Verification items for the finished model (mm, model axes). A direction names the side the tool comes from. Round coordinates to 2 decimals unless told otherwise and drop trailing zeros. Order: outer loops, then holes, each group sorted by start corner. A loop starts at its lowest first (then second) coordinate and runs counter-clockwise, first axis right, second up. Notation, with made-up numbers: (-39.75, 18) -> (-26.75, 18) arc R21 ccw to (-26.75, 22) -> close; hole circle Ø6 at (14, 53). An arc over 180 degrees is marked (long way). Return JSON: item names as keys, results as strings. Group by question number.
1) Tool access check on faces 1 (the flat face through (7, 0, 8)), 2 (the flat face through (-12.3, -3.7, 9)), 3 (the flat face through (-6, 3, 14)). Record the directions out of +Z, -Z, +X, -X, +Y, -Y that give a thin tool (end or side, any length) a straight path to the whole face; none if there is none.
2) Draft check along Y on faces 4 (the cylindrical face through (-4.769, -21.477, 6.902)), 5 (the cylindrical face through (-1.398, -6.297, 11.042)), 6 (the flat face through (-8.3, -16.2, 14)). Enter one of: pulls with the +Y half, pulls with the -Y half, needs draft (parallel to the pull), parting line crosses it, or undercut.
3) Section check A-A on x = 0. Enter the section's corners in (y, z).
4) Scan lines: L1, parallel to Y at x = 0, z = 10.7; L2, parallel to Y at x = 0, z = 2.5; L3, parallel to X at y = -9.5, z = 9.5. Record each from-to range of solid material in increasing order.
5) Depth check by flat-ended pin: pin 1 (3 mm diameter, centred on x = 1, z = 2, fed in from -Y); pin 2 (1 mm diameter, centred on x = -5.5, y = -12, fed in from +Z); pin 3 (4 mm diameter, centred on x = -2.5, y = -6, fed in from -Z). Enter the tip coordinate at first touch or a pass-through.
6) Section check C-C on z = 11.25. Enter the section's corners in (x, y).
7) Section check D-D on y = -14.5. Enter the section's corners in (x, z).
```python
from build123d import *

# Parameters (mm, degrees)
SKETCH_R        = 22
PAD_DEPTH       = 14
SKETCH001_R     = 18
POCKET_DEPTH    = 5
SKETCH002_R     = 12.6
PAD001_DEPTH    = 5
SKETCH003_R     = 6.45
POCKET001_DEPTH = 14.001
SKETCH004_R     = 16.2
POCKET002_DEPTH = 8


with BuildPart() as part:
    # Sketch → Pad (new body)
    with BuildSketch(Plane.XY):
        Circle(SKETCH_R)
    extrude(amount=PAD_DEPTH)

    # Sketch001 → Pocket (cut)
    with BuildSketch(Plane.XY.offset(14)):
        Circle(SKETCH001_R)
    extrude(amount=-POCKET_DEPTH, mode=Mode.SUBTRACT)

    # Sketch002 → Pad001 (new body)
    with BuildSketch(Plane.XY.offset(9)):
        Circle(SKETCH002_R)
    extrude(amount=PAD001_DEPTH)

    # Sketch003 → Pocket001 (cut, through all)
    with BuildSketch(Plane.XY.offset(14)):
        Circle(SKETCH003_R)
    extrude(amount=-POCKET001_DEPTH, mode=Mode.SUBTRACT)

    # Sketch004 → Pocket002 (cut)
    with BuildSketch(Plane(origin=(0, 0, 0), x_dir=(1, 0, 0), z_dir=(0, 0, -1))):
        Circle(SKETCH004_R)
    extrude(amount=-POCKET002_DEPTH, mode=Mode.SUBTRACT)


solid = part.part
```
Check result:
{
 "1": {"face 1": "-Z", "face 2": "+Z", "face 3": "+Z, +X, -X, +Y, -Y"},
 "2": {"face 4": "parting line crosses it", "face 5": "undercut", "face 6": "needs draft"},
 "3": {"outline": "(-22, 0) -> (-16.2, 0) -> (-16.2, 8) -> (-6.45, 8) -> (-6.45, 14) -> (-12.6, 14) -> (-12.6, 9) -> (-18, 9) -> (-18, 14) -> (-22, 14) -> close; (6.45, 8) -> (16.2, 8) -> (16.2, 0) -> (22, 0) -> (22, 14) -> (18, 14) -> (18, 9) -> (12.6, 9) -> (12.6, 14) -> (6.45, 14) -> close"},
 "4": {"L1": "-22 to -18, -12.6 to -6.45, 6.45 to 12.6, 18 to 22", "L2": "-22 to -16.2, 16.2 to 22", "L3": "-19.84 to -15.29, -8.28 to 8.28, 15.29 to 19.84"},
 "5": {"pin 1": "y = -22", "pin 2": "z = 9", "pin 3": "z = 8"},
 "6": {"outline": "circle Ø44 at (0, 0); circle Ø25.2 at (0, 0); hole circle Ø36 at (0, 0); hole circle Ø12.9 at (0, 0)"},
 "7": {"outline": "(-16.55, 0) -> (-7.22, 0) -> (-7.22, 8) -> (7.22, 8) -> (7.22, 0) -> (16.55, 0) -> (16.55, 14) -> (10.67, 14) -> (10.67, 9) -> (-10.67, 9) -> (-10.67, 14) -> (-16.55, 14) -> close"}
}
